Can you work these out from the model? Positions are in its coordinate system, mm. Give positions to 0.01 mm unless a question says otherwise; leave off trailing zeros. Answer as a JSON object with one key per item and string values.
```python
from build123d import *

# Parameters (mm, degrees)
F0_W     = 300
F0_H     = 300
F1_DEPTH = 30
F2_D     = 10
F3_R     = 25
F4_SIZE2 = 10
F4_SIZE  = 10


with BuildPart() as f1:
    # F0 (on Top) → F1 (new body)
    with BuildSketch(Plane.XY):
        with Locations((150, 150)):
            Rectangle(F0_W, F0_H)
    extrude(amount=F1_DEPTH)

    # F2 (through all)
    with Locations(Plane(origin=(0, 0, 0), x_dir=(1, 0, 0), z_dir=(0, 0, -1))):
        with Locations((275, -275), (25, -275), (275, -25), (25, -25)):
            Hole(F2_D / 2)

    # F3
    f3_edges = [f1.edges().sort_by_distance(p)[0] for p in [
        (0, 300, 15),
        (0, 0, 15),
        (300, 0, 15),
        (300, 300, 15),
    ]]
    fillet(f3_edges, radius=F3_R)

    # F4
    f4_edges = [f1.edges().sort_by_distance(p)[0] for p in [
        (0, 150, 30),
    ]]
    chamfer(f4_edges, length=F4_SIZE, length2=F4_SIZE2)


solid = f1.part
```
1. Will these pins go through, and if not, where does the flat tip stop? pin 1 Ø6 at (x, y) = (275, 275) entering from -Z; pin 2 Ø1.5 at (x, z) = (46, 23) entering from +Y; pin 3 Ø13 at (x, y) = (275, 25) entering from +Z; pin 4 Ø6 at (x, z) = (191, 26) entering from +Y.
Worked answers:
{"pin 1": "through", "pin 2": "y = 297.75", "pin 3": "z = 30", "pin 4": "y = 297"}
2. Please list where these lines run through material, in increasing order: L1, parallel to X at y = 275, z = 19.5; L2, parallel to Y at x = 25, z = 20.25.
Worked answers:
{"L1": "0 to 20, 30 to 270, 280 to 300", "L2": "0.25 to 20, 30 to 270, 280 to 299.75"}
3. If we mould it in two halves opening along Y, with no side actions, what happens to faces 1 (the face through (270.381, 26.915, 15.21)), 2 (the face through (288.45, 11.84, 26.18)), 3 (the face through (148, 300, 10))? For each: +Y half, -Y half, draft (parallel to the pull), parting line (faces both ways), or undercut.
Worked answers:
{"face 1": "undercut", "face 2": "-Y half", "face 3": "+Y half"}
